The model under review builds one solid part; all positions refer to its coordinate system, in mm. Face numbers are marked on the shaded views. A direction names the side the tool comes from. Round coordinates to 2 decimals unless told otherwise and drop trailing zeros. Loops run counter-clockwise (first coordinate to the right, second up) from the corner with the lowest first, then second, coordinate; pieces in that order, holes last. Notation, with made-up numbers: (59.25, 13) - (83.25, 13) arc R20 cw to (83.25, 33) - close; hole circle Ø7 at (-40, 34). An arc over 180 degrees is marked (long way). Answer as CSV lines item,"result".
Autodesk Inventor part; units mm, degrees
ref_plane "YZ Plane" through (0, 0, 0) normal (1, 0, 0) x (0, 1, 0)
ref_plane "XZ Plane" through (0, 0, 0) normal (0, 1, 0) x (-1, 0, 0)
ref_plane "XY Plane" through (0, 0, 0) normal (0, 0, 1) x (1, 0, 0)
sketch "Skizze1" plane through (0, 0, 0) normal (0, 0, 1) x (1, 0, 0)
  circle A0 centre (0, 0) radius 3.5
  dimension "d0" = 7
extrude "Extrusion1" add sketch "Skizze1" along normal blind 7
sketch "Skizze2" plane through (0, 0, 0) normal (0, 0, -1) x (-1, 0, 0)
  line L0 (-7.5, 7.5) -> (7.5, 7.5)
  line L1 (7.5, 7.5) -> (7.5, -7.5)
  line L2 (7.5, -7.5) -> (-7.5, -7.5)
  line L3 (-7.5, -7.5) -> (-7.5, 7.5)
  line L4 (-7.5, 7.5) -> (7.5, -7.5) construction
  line L5 (7.5, 7.5) -> (-7.5, -7.5) construction
  point P0 (0, 0)
  dimension "d3" = 15
  dimension "d4" = 15
extrude "Extrusion2" add sketch "Skizze2" along normal blind 6.8
sketch "Skizze3" plane through (0, 0, -6.8) normal (0, 0, -1) x (-1, 0, 0)
  line L0 (-8.6809, 12.15) -> (8.9191, 12.15)
  line L1 (8.9191, 12.15) -> (8.9191, -17.45)
  line L2 (8.9191, -17.45) -> (-8.6809, -17.45)
  line L3 (-8.6809, -17.45) -> (-8.6809, 12.15)
  line L4 (7.5, 7.5) -> (-7.5, 7.5)
  point P0 (0, 0)
  dimension "d7" = 17.6
  dimension "d8" = 29.6
  dimension "d9" = 4.65
extrude "Extrusion3" add sketch "Skizze3" along normal blind 2
sketch "Skizze4" plane through (0, 0, 7) normal (0, 0, 1) x (1, 0, 0)
  circle A0 centre (0, 0) radius 3
  dimension "d12" = 6
extrude "Extrusion4" add sketch "Skizze4" along normal blind 13.5
sketch "Skizze5" plane through (0, 0, 20.5) normal (0, 0, 1) x (1, 0, 0)
  line L0 (-8.9965, 8.617) -> (9.175, 8.617)
  line L1 (9.175, 8.617) -> (9.175, -9.4653)
  line L2 (9.175, -9.4653) -> (-8.9965, -9.4653)
  line L3 (-8.9965, -9.4653) -> (-8.9965, 8.617)
  point P0 (0, 0)
extrude "Extrusion5" cut sketch "Skizze5" against normal blind 5
equation "\"d4\" = d3"
properties part number "encoder"
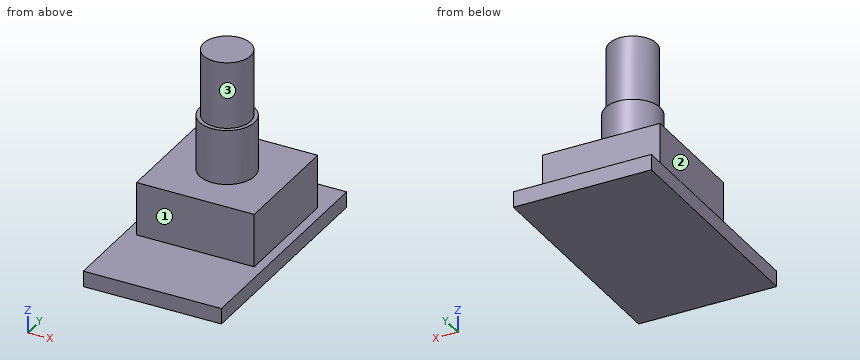
1. Tool access review of the marked faces 1, 2 and 3: name each direction out of +Z, -Z, +X, -X, +Y, -Y from which nothing blocks a thin tool from reaching the whole face with its end or side.
Numbers:
face 1,"+Z, +X, -X, -Y"
face 2,"+Z, -X, +Y, -Y"
face 3,"+Z"
2. Take a section at A-A (x = 0). State the section outline as (y, z) points, plus the area to 3 significant figures.
Numbers:
outline,"(-17.45, -8.8) - (12.15, -8.8) - (12.15, -6.8) - (7.5, -6.8) - (7.5, 0) - (3.5, 0) - (3.5, 7) - (3, 7) - (3, 15.5) - (-3, 15.5) - (-3, 7) - (-3.5, 7) - (-3.5, 0) - (-7.5, 0) - (-7.5, -6.8) - (-17.45, -6.8) - close"
area,"261 mm²"
3. Take a section at B-B (y = 0). State the section outline as (x, z) points, plus the area to 3 significant figures.
Numbers:
outline,"(-8.92, -8.8) - (8.68, -8.8) - (8.68, -6.8) - (7.5, -6.8) - (7.5, 0) - (3.5, 0) - (3.5, 7) - (3, 7) - (3, 15.5) - (-3, 15.5) - (-3, 7) - (-3.5, 7) - (-3.5, 0) - (-7.5, 0) - (-7.5, -6.8) - (-8.92, -6.8) - close"
area,"237 mm²"
4. Wall thickness on probe 1 along Z at (x, y) = (-6, -16); probe 2 along Y at (x, z) = (-2.25, -1.25); probe 3 along Z at (x, y) = (-1.75, 6.25): over which ranges is each line inside the solid? List them lowest first.
Numbers:
probe 1,"z = -8.8 to -6.8"
probe 2,"y = -7.5 to 7.5"
probe 3,"z = -8.8 to 0"
5. Take a section at D-D (x = 5.25). State the section outline as (y, z) points.
Numbers:
outline,"(-17.45, -8.8) - (12.15, -8.8) - (12.15, -6.8) - (7.5, -6.8) - (7.5, 0) - (-7.5, 0) - (-7.5, -6.8) - (-17.45, -6.8) - close"
6. Clearance check with flat-ended pins moving along their axes: pin 1 (10 mm diameter, centred on x = -6.5, y = -7.5, fed in from +Z); pin 2 (6 mm diameter, centred on y = -13, z = -2.5, fed in from -X); pin 3 (3 mm diameter, centred on x = 4.5, z = -3, fed in from +Y); pin 4 (2 mm diameter, centred on x = 3.5, z = -3, fed in from -Y). State where each tip first meets the part, or that it passes through.
Numbers:
pin 1,"stops at z = 0"
pin 2,"passes through"
pin 3,"stops at y = 7.5"
pin 4,"stops at y = -7.5"
7. Take a section at C-C (z = -0.75). State the section outline as (x, y) points.
Numbers:
outline,"(-7.5, -7.5) - (7.5, -7.5) - (7.5, 7.5) - (-7.5, 7.5) - close"
